Could you check a few things on this model? Use its own coordinates, in mm. Face numbers are marked on the shaded views. A direction names the side the tool comes from. Give positions to 0.01 mm unless a question says otherwise; leave off trailing zeros. Loops run counter-clockwise (first coordinate to the right, second up) from the corner with the lowest first, then second, coordinate; pieces in that order, holes last. Notation, with made-up numbers: (75, 0.25) -> (118, 0.25) arc R22 ccw to (118, 33.25) -> close; hole circle Ø3 at (66, 0.25). An arc over 180 degrees is marked (long way). Write each question's results on one line, items separated by ' | '. Start each with the question number.
Q1. We'd pull the mould along X, two halves only. Please class the marked faces 6, 7 and 8: released by +X, released by -X, zero draft, split by the parting line, or undercut.
Q2. Which directions (+Z, -Z, +X, -X, +Y, -Y) give clear straight access to the entire face, cutting with the end or side of a thin tool? Please do the marked faces 1, 2, 3, 4 and 5.
Q3. Will these pins go through, and if not, where does the flat tip stop? P1, Ø9.5, axis at x = -2, z = 1, coming from the +Y side; P2, Ø12.5, axis at x = -8.5, y = 23.5, coming from the -Z side; P3, Ø6.5, axis at x = -0.5, z = -8.5, coming from the +Y side.
Q4. If I drill on line 1 along Z through (x, y) = (-11.5, 14); line 2 along X through (y, z) = (22, 4); line 3 along X through (y, z) = (14, 0.25), over which ranges is the centre line in solid material (lowest first)?
Q5. If we section it at D-D, the plane y = 27.5: List the corners of the cut face in (x, z) for me.
Q6. If we section it at B-B, the plane z = 0: List the corners of the cut face in (x, y) for me, plus the area to 3 significant figures.
Q7. If we section it at C-C, the plane x = 0: List the corners of the cut face in (y, z) for me, plus the area to 3 significant figures.
Q8. If we section it at A-A, the plane y = 19.5: List the corners of the cut face in (x, z) for me.
from build123d import *

# Parameters (mm, degrees)
SKETCH1_R           = 12.5
BOSS_EXTRUDE1_DEPTH = 7.5
SKETCH2_W           = 35
SKETCH2_H           = 8.580767914
BOSS_EXTRUDE2_DEPTH = 25
SKETCH3_W           = 25
SKETCH3_H           = 8.580767914
CUT_EXTRUDE1_DEPTH  = 20
SKETCH4_R           = 2.5
BOSS_EXTRUDE3_DEPTH = 3.75
SKETCH5_R           = 2.5
BOSS_EXTRUDE4_DEPTH = 3.75
CHAMFER1_SIZE       = 5
CHAMFER2_SIZE       = 5


with BuildPart() as part:
    # Sketch1 → Boss-Extrude1 (new body)
    with BuildSketch(Plane(origin=(0, 0, 0), x_dir=(1, 0, 0), z_dir=(0, 1, 0))):
        Circle(SKETCH1_R)
    extrude(amount=BOSS_EXTRUDE1_DEPTH)

    # Sketch2 → Boss-Extrude2 (add)
    with BuildSketch(Plane(origin=(0, 7.5, 0), x_dir=(1, 0, 0), z_dir=(0, 1, 0))):
        Rectangle(SKETCH2_W, SKETCH2_H)
    extrude(amount=BOSS_EXTRUDE2_DEPTH)

    # Sketch3 → Cut-Extrude1 (cut)
    with BuildSketch(Plane(origin=(0, 32.5, 0), x_dir=(1, 0, 0), z_dir=(0, 1, 0))):
        Rectangle(SKETCH3_W, SKETCH3_H)
    extrude(amount=-CUT_EXTRUDE1_DEPTH, mode=Mode.SUBTRACT)

    # Sketch4 → Boss-Extrude3 (add)
    with BuildSketch(Plane(origin=(-12.5, 0, 0), x_dir=(0, 0, -1), z_dir=(1, 0, 0))):
        with Locations((0, 27.5)):
            Circle(SKETCH4_R)
    extrude(amount=BOSS_EXTRUDE3_DEPTH)

    # Sketch5 → Boss-Extrude4 (add)
    with BuildSketch(Plane.ZY.offset(-12.5)):
        with Locations((0, 27.5)):
            Circle(SKETCH5_R)
    extrude(amount=BOSS_EXTRUDE4_DEPTH)

    # Chamfer1
    chamfer1_edges = [part.edges().sort_by_distance(p)[0] for p in [
        (-12.5, 12.5, 0),
    ]]
    chamfer(chamfer1_edges, length=CHAMFER1_SIZE)

    # Chamfer2
    chamfer2_edges = [part.edges().sort_by_distance(p)[0] for p in [
        (12.5, 12.5, 0),
    ]]
    chamfer(chamfer2_edges, length=CHAMFER2_SIZE)


solid = part.part
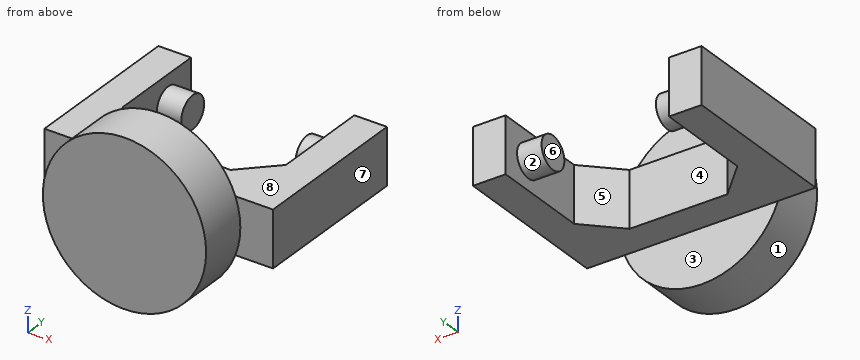
Final values:
1) face 6: undercut | face 7: released by +X | face 8: zero draft
2) face 1: -Y | face 2: none | face 3: -Z, +X, -X, +Y | face 4: +Z, -Z, +Y | face 5: +Z, -Z
3) P1: stops at y = 12.5 | P2: stops at z = -4.29 | P3: stops at y = 7.5
4) line 1: z = -4.29 to 4.29 | line 2: x = -17.5 to -12.5, 12.5 to 17.5 | line 3: x = -17.5 to -9, 9 to 17.5
5) outline: (-17.5, -4.29) -> (-12.5, -4.29) -> (-12.5, -2.5) -> (-8.75, -2.5) -> (-8.75, 2.5) -> (-12.5, 2.5) -> (-12.5, 4.29) -> (-17.5, 4.29) -> close; (8.75, -2.5) -> (12.5, -2.5) -> (12.5, -4.29) -> (17.5, -4.29) -> (17.5, 4.29) -> (12.5, 4.29) -> (12.5, 2.5) -> (8.75, 2.5) -> close
6) outline: (-17.5, 7.5) -> (-12.5, 7.5) -> (-12.5, 0) -> (12.5, 0) -> (12.5, 7.5) -> (17.5, 7.5) -> (17.5, 32.5) -> (12.5, 32.5) -> (12.5, 30) -> (8.75, 30) -> (8.75, 25) -> (12.5, 25) -> (12.5, 17.5) -> (7.5, 12.5) -> (-7.5, 12.5) -> (-12.5, 17.5) -> (-12.5, 25) -> (-8.75, 25) -> (-8.75, 30) -> (-12.5, 30) -> (-12.5, 32.5) -> (-17.5, 32.5) -> close | area: 625 mm²
7) outline: (0, -12.5) -> (7.5, -12.5) -> (7.5, -4.29) -> (12.5, -4.29) -> (12.5, 4.29) -> (7.5, 4.29) -> (7.5, 12.5) -> (0, 12.5) -> close | area: 230 mm²
8) outline: (-17.5, -4.29) -> (-12.5, -4.29) -> (-12.5, 4.29) -> (-17.5, 4.29) -> close; (12.5, -4.29) -> (17.5, -4.29) -> (17.5, 4.29) -> (12.5, 4.29) -> close
